Input: part model. Units: mm. Frame: model coordinates. Coordinates: 2 decimals unless noted, no trailing zeros. Write each loop counter-clockwise with the first axis right and the second up, starting at its lowest first coordinate (ties: lowest second). Pieces come first, ordered by that corner, then holes. Notation, with made-up numbers: (64, 87.5) - (93, 87.5) arc R18 ccw to (93, 118.5) - close; hole circle Ø8 at (28, 24). An arc over 180 degrees is marked (long way). Use CSV: the item, a comma, the result in double quotes.
```python
from build123d import *

# Parameters (mm, degrees)
SKETCH_1_W          = 235
SKETCH_1_H          = 250
EXTRUDE_1_DEPTH     = 3
SKETCH_2_W          = 107
SKETCH_2_H          = 72
CUT_EXTRUDE_1_DEPTH = 172.581613234
SKETCH_3_R          = 2.1
CUT_EXTRUDE_2_DEPTH = 10
SKETCH_4_R          = 1.6
CUT_EXTRUDE_3_DEPTH = 3
CUT_EXTRUDE_4_DEPTH = 172.581613234
SKETCH_6_R          = 2.1
CUT_EXTRUDE_5_DEPTH = 3
FILLET_1_R          = 5
FILLET_2_R          = 3


with BuildPart() as part:
    # 草图1 → 凸台-拉伸1 (new body)
    with BuildSketch(Plane.XY):
        Rectangle(SKETCH_1_W, SKETCH_1_H)
    extrude(amount=EXTRUDE_1_DEPTH)

    # 草图2 → 切除-拉伸1 (cut, through all)
    with BuildSketch(Plane.XY.offset(3)):
        with Locations((64, 0)):
            Rectangle(SKETCH_2_W, SKETCH_2_H)
    extrude(amount=-CUT_EXTRUDE_1_DEPTH, mode=Mode.SUBTRACT)

    # 草图3 → 切除-拉伸2 (cut)
    with BuildSketch(Plane.XY.offset(3)):
        with Locations((-94.5, 98)):
            Circle(SKETCH_3_R)
        with Locations((-24.5, 98)):
            Circle(SKETCH_3_R)
    cut_extrude_2 = extrude(amount=-CUT_EXTRUDE_2_DEPTH, mode=Mode.SUBTRACT)

    # 镜向1: 切除-拉伸2 across plane
    add(cut_extrude_2.mirror(Plane.ZX), mode=Mode.SUBTRACT)

    # 草图4 → 切除-拉伸3 (cut)
    with BuildSketch(Plane.XY.offset(3)):
        with Locations((108.5, 48)):
            Circle(SKETCH_4_R)
        with Locations((-1.5, 48)):
            Circle(SKETCH_4_R)
        with Locations((108.5, -48)):
            Circle(SKETCH_4_R)
        with Locations((-1.5, -48)):
            Circle(SKETCH_4_R)
    extrude(amount=-CUT_EXTRUDE_3_DEPTH, mode=Mode.SUBTRACT)

    # 草图5 → 切除-拉伸4 (cut, through all)
    with BuildSketch(Plane.XY.offset(3)):
        Polygon((117.5, 125), (27.5, 125), (-4.025914193, 125), (-19.025914193, 125), (-19.025914193, 105.446897357), (-4.496566438, 105.446897357), (-4.496879266, 85.446897359), (27.5, 85), (27.5, 75), (67.5, 75), (67.5, 65), (117.5, 65), align=None)
    cut_extrude_4 = extrude(amount=-CUT_EXTRUDE_4_DEPTH, mode=Mode.SUBTRACT)

    # 镜向2: 切除-拉伸4 across plane
    add(cut_extrude_4.mirror(Plane.ZX), mode=Mode.SUBTRACT)

    # 草图6 → 切除-拉伸5 (cut)
    with BuildSketch(Plane.XY.offset(3)):
        with Locations((-82, -116)):
            Circle(SKETCH_6_R)
        with Locations((-37, -116)):
            Circle(SKETCH_6_R)
    cut_extrude_5 = extrude(amount=-CUT_EXTRUDE_5_DEPTH, mode=Mode.SUBTRACT)

    # 镜向3: 切除-拉伸5 across plane
    add(cut_extrude_5.mirror(Plane.ZX), mode=Mode.SUBTRACT)

    # 圆角1
    fillet_1_edges = [part.edges().sort_by_distance(p)[0] for p in [
        (117.5, -65, 1.5),
        (-19.025914193, -105.446897357, 1.5),
        (-4.496879266, -85.446897359, 1.5),
        (27.5, -75, 1.5),
        (67.5, -65, 1.5),
        (10.5, -36, 1.5),
        (10.5, 36, 1.5),
        (117.5, 36, 1.5),
        (117.5, -36, 1.5),
        (117.5, 65, 1.5),
        (67.5, 65, 1.5),
        (27.5, 75, 1.5),
        (-4.496879266, 85.446897359, 1.5),
        (-19.025914193, 105.446897357, 1.5),
    ]]
    fillet(fillet_1_edges, radius=FILLET_1_R)

    # 圆角2
    fillet_2_edges = [part.edges().sort_by_distance(p)[0] for p in [
        (-19.025914193, -125, 1.5),
        (-4.496566438, -105.446897357, 1.5),
        (27.5, -85, 1.5),
        (67.5, -75, 1.5),
        (-117.5, -125, 1.5),
        (-117.5, 125, 1.5),
        (67.5, 75, 1.5),
        (27.5, 85, 1.5),
        (-4.496566438, 105.446897357, 1.5),
        (-19.025914193, 125, 1.5),
    ]]
    fillet(fillet_2_edges, radius=FILLET_2_R)


solid = part.part
```
(1) Cut plane A-A on z = 0.85. State how many separate pieces and enclosed holes the cut face has, and give its area (3 significant figures).
Check values:
separate pieces,"1"
enclosed holes,"12"
area,"37,800 mm^2"
(2) Ray query, probe 1 along X at (y, z) = (-98, 1.65); probe 2 along Y at (x, z) = (-37, 1.3); probe 3 along Y at (x, z) = (-1.5, 1.45). Return the intervals inside material, ascending. Write a range as from..to.
Check values:
probe 1,"-117.5..-96.6, -92.4..-26.6, -22.4..-4.5"
probe 2,"-125..-118.1, -113.9..113.9, 118.1..125"
probe 3,"-85.8..-49.6, -46.4..46.4, 49.6..85.8"
(3) Cut plane B-B on y = 21. Return loops of the section in (x, z), and give its area (3 significant figures).
Check values:
outline,"(-117.5, 0) - (10.5, 0) - (10.5, 3) - (-117.5, 3) - close"
area,"384 mm^2"
(4) Pin query (flat end, axial travel): pin 1 Ø1.5 at (x, z) = (83, 2.5) entering from +Y; pin 2 Ø1 at (x, z) = (89, 0.5) entering from -Y. Return the tip coordinate at first contact, or that it passes through.
Check values:
pin 1,"y = 65"
pin 2,"y = -65"
